from build123d import *

# Parameters (mm, degrees)
FILLET1_R      = 0.79375
CHAMFER1_SIZE  = 0.79375
CHAMFER1_SIZE2 = 1.374815329


with BuildPart() as part:
    # Sketch1 → Revolve1 (revolve)
    with BuildSketch(Plane.XY):
        Polygon((0, 0), (-9.398, 0), (-9.398, 1.5875), (-7.62, 4.445), (-7.62, 7.62), (-9.398, 7.62), (-9.398, 12.7), (0, 12.7), align=None)
    revolve(axis=Axis((0, 0, 0), (0, 1, 0)))

    # Fillet1
    fillet1_edges = [part.edges().sort_by_distance(p)[0] for p in [
        (9.398, 0, 0),
    ]]
    fillet(fillet1_edges, radius=FILLET1_R)

    # Chamfer1
    chamfer1_edges = [part.edges().sort_by_distance(p)[0] for p in [
        (9.398, 12.7, 0),
    ]]
    chamfer1_side = [part.faces().sort_by_distance(p)[0] for p in [
        (0, 12.7, 0),
    ]]
    chamfer(chamfer1_edges, length=CHAMFER1_SIZE, length2=CHAMFER1_SIZE2, reference=chamfer1_side[0])


solid = part.part
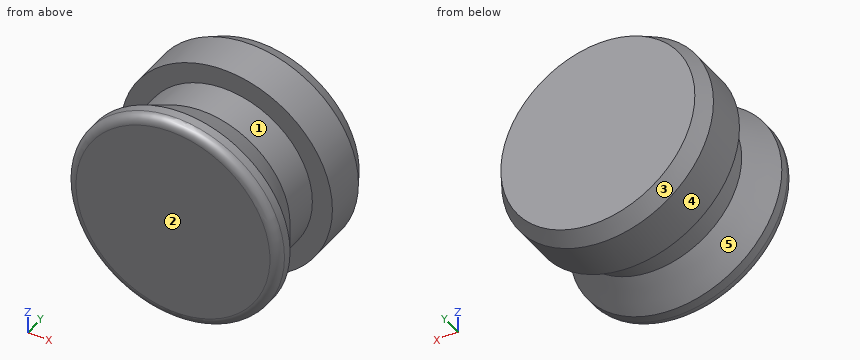
Geometry: final body of the model. Coordinates: model frame, mm. Face numbers are marked on the shaded views. A direction names the side the tool comes from. Give positions to 0.01 mm unless a question says otherwise; leave off trailing zeros. Order: outer loops, then holes, each group sorted by start corner. A loop starts at its lowest first (then second) coordinate and runs counter-clockwise, first axis right, second up. Notation, with made-up numbers: (46.5, 3) - (77.5, 3) arc R28 cw to (77.5, 23) - close; hole circle Ø2 at (-31.5, -10). An arc over 180 degrees is marked (long way). Use CSV: the item, a comma, the result in double quotes.
1. Section query C-C (y = 8). Output: boundary loops of the cut face in (x, z).
Answers below:
outline,"circle Ø18.8 at (0, 0)"
2. Section query B-B (z = 0). Output: boundary loops of the cut face in (x, y) (1 decimal), plus the area to 3 significant figures.
Answers below:
outline,"(-9.4, 0.8) arc R0.8 ccw to (-8.6, 0) - (8.6, 0) arc R0.8 ccw to (9.4, 0.8) - (9.4, 1.6) - (7.6, 4.4) - (7.6, 7.6) - (9.4, 7.6) - (9.4, 11.3) - (8.6, 12.7) - (-8.6, 12.7) - (-9.4, 11.3) - (-9.4, 7.6) - (-7.6, 7.6) - (-7.6, 4.4) - (-9.4, 1.6) - close"
area,"221 mm2"
3. Contact query for flat-ended pins moving along their axis: pin 1 (5.5 mm diameter, centred on x = -3.5, z = 2, fed in from -Y); pin 2 (2 mm diameter, centred on x = -3.5, y = 3, fed in from -Z); pin 3 (2 mm diameter, centred on x = -1.5, y = 5.5, fed in from +Z); pin 4 (5 mm diameter, centred on x = 6.5, y = 6.5, fed in from -Z). Output: stop coordinate, or through.
Answers below:
pin 1,"y = 0"
pin 2,"z = -8.55"
pin 3,"z = 7.6"
pin 4,"z = -8.37"
4. Section query D-D (y = 3.5). Output: boundary loops of the cut face in (x, z).
Answers below:
outline,"circle Ø16.42 at (0, 0)"
5. Mould query, pull axis Y, two halves, no side actions, for the marked faces 3, 4 and 5. Classes: +Y half, -Y half, draft (parallel to the pull), parting line (faces both ways), or undercut.
Answers below:
face 3,"+Y half"
face 4,"draft"
face 5,"undercut"
6. Material intervals for line 1 along X through (y, z) = (10.25, -0.25); line 2 along X through (y, z) = (11.25, -6.75); line 3 along Z through (x, y) = (2.25, 4), sorted ascending. Write a range as from..to.
Answers below:
line 1,"-9.39..9.39"
line 2,"-6.54..6.54"
line 3,"-7.57..7.57"
7. Section query A-A (x = 0). Output: boundary loops of the cut face in (y, z) (1 decimal).
Answers below:
outline,"(0, -8.6) arc R0.8 ccw to (0.8, -9.4) - (1.6, -9.4) - (4.4, -7.6) - (7.6, -7.6) - (7.6, -9.4) - (11.3, -9.4) - (12.7, -8.6) - (12.7, 8.6) - (11.3, 9.4) - (7.6, 9.4) - (7.6, 7.6) - (4.4, 7.6) - (1.6, 9.4) - (0.8, 9.4) arc R0.8 ccw to (0, 8.6) - close"
8. Access query for the marked faces 1 and 2. Directions: +Z, -Z, +X, -X, +Y, -Y. A direction counts if a zero-diameter tool reaches every point of the face in a straight line with its end or side. Return the directions, or none.
Answers below:
face 1,"none"
face 2,"+Z, -Z, +X, -X, -Y"
